Part model, mm, in its own coordinate system. A direction names the side the tool comes from. Give positions to 0.01 mm unless a question says otherwise; leave off trailing zeros. Answer as CSV lines item,"result". Start each with the question number.
1) Pin check, flat tips, straight feed: pin 1 Ø5 at (x, z) = (51.5, -35.5) entering from +Y; pin 2 Ø5 at (x, y) = (50, 102.5) entering from +Z; pin 3 Ø25 at (x, y) = (33, 62.5) entering from -Z. Stop position of each tip, or through.
2) Wall check: line 1 along X through (y, z) = (31, -4); line 2 along Z through (x, y) = (58.5, 97.5); line 3 along Y through (x, z) = (9, -16.5). Give the ranges that are in metal, low to high. Write a range as from..to.
3) Tool access for faces 1 (the flat face through (112.5, 45, -14)), 2 (the flat face through (57, 77, -19.295)): list every direction of +Z, -Z, +X, -X, +Y, -Y with a clear straight run to the whole face (end or side of a thin tool).
Autodesk Inventor part; units mm, degrees
ref_plane "Work Plane4" through (0, 100, 0) normal (0, 0.7071068, 0.7071068) x (1, 0, 0)
ref_plane "YZ Plane" through (0, 0, 0) normal (1, 0, 0) x (0, 1, 0)
ref_plane "XZ Plane" through (0, 0, 0) normal (0, 1, 0) x (-1, 0, 0)
sketch "Sketch1" plane through (0, 0, 0) normal (0, 0, 1) x (1, 0, 0)
  arc A0 (12.7973, -6.8176) -> (-12.597, -7.1809) centre (0, 0) ccw
  arc A1 (50.4829, -6.2785) -> (26.2017, -6.6259) centre (38.25, 0) ccw
  arc A2 (85.5853, -5.7763) -> (63.5844, -6.091) centre (74.5, 0) ccw
  arc A3 (117.8988, -5.314) -> (98.5072, -5.5914) centre (108.125, 0) ccw
  arc A4 (147.9764, -4.8837) -> (130.6669, -5.1313) centre (139.25, 0) ccw
  arc A5 (177.1345, -4.4665) -> (160.4967, -4.7045) centre (168.75, 0) ccw
  line L0 (-20, 20) -> (188.75, 20)
  line L1 (188.75, 20) -> (188.75, -4.3003)
  line L2 (-20, 20) -> (-20, -7.2868)
  line L3 (-20, -7.2868) -> (188.75, -4.3003)
  dimension "d0" = 29
  dimension "d1" = 27.5
  dimension "d2" = 25
  dimension "d3" = 22.25
  dimension "d4" = 20
  dimension "d5" = 19
  dimension "d6" = 38.25
  dimension "d7" = 36.25
  dimension "d8" = 33.625
  dimension "d9" = 31.125
  dimension "d10" = 29.5
  dimension "d11" = 0
  dimension "d12" = 0
  dimension "d13" = 0
  dimension "d14" = 0
  dimension "d15" = 0
  dimension "d20" = 20
  dimension "d22" = 20
  dimension "d23" = 20
  dimension "d24" = 7
  dimension "d25" = 4.586
sketch "Sketch4" plane through (0, 0, 0) normal (1, 0, 0) x (0, 1, 0)
  line L0 (0, 0) -> (29.9033, -29.9033)
  line L1 (0, 5.9807) -> (0, -35.884)
  point P0 (100, 0)
  dimension "d51" = 45
  dimension "d53" = 0
  dimension "d55" = 29.9033
  dimension "d98" = 100
ref_plane "Work Plane4" through (0, 100, 0) normal (0, 0.7071068, 0.7071068) x (1, 0, 0)
ref_plane "Work Plane3" through (-10, 0, 0) normal (0, 0.7071068, 0.7071068) x (1, 0, 0)
sketch "Sketch5" plane through (-10, 0, 0) normal (0, 0.7071068, 0.7071068) x (1, 0, 0)
  arc A0 (42.7973, 0.4692) -> (17.403, 0.1059) centre (30, 7.2868) ccw
  arc A1 (80.4829, 1.0084) -> (56.2017, 0.661) centre (68.25, 7.2868) ccw
  arc A2 (115.5853, 1.5106) -> (93.5844, 1.1958) centre (104.5, 7.2868) ccw
  arc A3 (147.8988, 1.9729) -> (128.5072, 1.6954) centre (138.125, 7.2868) ccw
  arc A4 (177.9764, 2.4032) -> (160.6669, 2.1555) centre (169.25, 7.2868) ccw
  arc A5 (207.1345, 2.8203) -> (190.4967, 2.5823) centre (198.75, 7.2868) ccw
  line L0 (10, 27.2868) -> (218.75, 27.2868)
  line L1 (218.75, 27.2868) -> (218.75, 2.9865)
  line L2 (10, 27.2868) -> (10, 0)
  line L3 (10, 0) -> (17.403, 0.1059)
  line L4 (42.7973, 0.4692) -> (56.2017, 0.661)
  line L5 (80.4829, 1.0084) -> (93.5844, 1.1958)
  line L6 (115.5853, 1.5106) -> (128.5072, 1.6954)
  line L7 (207.1345, 2.8203) -> (218.75, 2.9865)
  line L8 (147.8988, 1.9729) -> (160.6669, 2.1555)
  line L9 (177.9764, 2.4032) -> (190.4967, 2.5823)
  dimension "d56" = 29
  dimension "d57" = 27.5
  dimension "d58" = 25
  dimension "d59" = 22.25
  dimension "d60" = 20
  dimension "d61" = 19
  dimension "d62" = 38.25
  dimension "d63" = 36.25
  dimension "d64" = 33.625
  dimension "d65" = 31.125
  dimension "d66" = 29.5
  dimension "d67" = 0
  dimension "d68" = 0
  dimension "d69" = 0
  dimension "d70" = 0
  dimension "d71" = 0
  dimension "d72" = 20
  dimension "d73" = 20
  dimension "d74" = 20
sketch "Sketch6" plane through (0, 100, 0) normal (0, 0.7071068, 0.7071068) x (1, 0, 0)
  arc A0 (32.7973, 0.4692) -> (7.403, 0.1059) centre (20, 7.2868) ccw
  arc A1 (70.4829, 1.0084) -> (46.2017, 0.661) centre (58.25, 7.2868) ccw
  arc A2 (105.5853, 1.5106) -> (83.5844, 1.1958) centre (94.5, 7.2868) ccw
  arc A3 (137.8988, 1.9729) -> (118.5072, 1.6954) centre (128.125, 7.2868) ccw
  arc A4 (167.9764, 2.4032) -> (150.6669, 2.1555) centre (159.25, 7.2868) ccw
  arc A5 (197.1345, 2.8203) -> (180.4967, 2.5823) centre (188.75, 7.2868) ccw
  line L0 (0, 27.2868) -> (208.75, 27.2868)
  line L1 (208.75, 27.2868) -> (208.75, 2.9865)
  line L2 (0, 27.2868) -> (0, 0)
  line L3 (0, 0) -> (7.403, 0.1059)
  line L4 (32.7973, 0.4692) -> (46.2017, 0.661)
  line L5 (70.4829, 1.0084) -> (83.5844, 1.1958)
  line L6 (105.5853, 1.5106) -> (118.5072, 1.6954)
  line L7 (137.8988, 1.9729) -> (150.6669, 2.1555)
  line L8 (167.9764, 2.4032) -> (180.4967, 2.5823)
  line L9 (197.1345, 2.8203) -> (208.75, 2.9865)
  point P0 (0, -70.7107)
  dimension "d77" = 29
  dimension "d78" = 27.5
  dimension "d79" = 25
  dimension "d80" = 22.25
  dimension "d81" = 20
  dimension "d82" = 19
  dimension "d83" = 38.25
  dimension "d84" = 36.25
  dimension "d85" = 33.625
  dimension "d86" = 31.125
  dimension "d87" = 29.5
  dimension "d88" = 0
  dimension "d89" = 0
  dimension "d90" = 0
  dimension "d91" = 0
  dimension "d92" = 0
  dimension "d93" = 20
  dimension "d94" = 20
  dimension "d95" = 20
loft "Loft1" add profiles "Sketch6", "Sketch5"
sketch "Sketch7" plane through (0, 0, 0) normal (0, 1, 0) x (-1, 0, 0)
  line L0 (0, 0) -> (0, -19.2947)
  line L1 (0, -19.2947) -> (-208.75, -19.2947)
  line L2 (-208.75, -19.2947) -> (-208.75, -2.1118)
  line L3 (-208.75, -2.1118) -> (-197.1345, -1.9943)
  ellipse E0 centre (-188.75, -5.1526) end of major axis (-198.25, -5.1526) minor radius 6.7175 (-197.1345, -1.9943) -> (-180.4967, -1.826) ccw
  line L4 (-180.4967, -1.826) -> (-167.9764, -1.6993)
  ellipse E1 centre (-159.25, -5.1526) end of major axis (-169.25, -5.1526) minor radius 7.0711 (-167.9764, -1.6993) -> (-150.6669, -1.5242) ccw
  line L5 (-150.6669, -1.5242) -> (-137.8988, -1.395)
  ellipse E2 centre (-128.125, -5.1526) end of major axis (-139.25, -5.1526) minor radius 7.8666 (-137.8988, -1.395) -> (-118.5072, -1.1989) ccw
  line L6 (-118.5072, -1.1989) -> (-105.5853, -1.0681)
  ellipse E3 centre (-94.5, -5.1526) end of major axis (-107, -5.1526) minor radius 8.8388 (-105.5853, -1.0681) -> (-83.5844, -0.8456) ccw
  line L7 (-83.5844, -0.8456) -> (-70.4829, -0.713)
  ellipse E4 centre (-58.25, -5.1526) end of major axis (-72, -5.1526) minor radius 9.7227 (-70.4829, -0.713) -> (-46.2017, -0.4674) ccw
  line L8 (-46.2017, -0.4674) -> (-32.7973, -0.3318)
  ellipse E5 centre (-20, -5.1526) end of major axis (-34.5, -5.1526) minor radius 10.253 (-32.7973, -0.3318) -> (-7.403, -0.0749) ccw
  line L9 (-7.403, -0.0749) -> (0, 0)
  line L10 (0, 0) -> (0, -19.2947)
  line L11 (0, -19.2947) -> (-208.75, -19.2947)
  line L12 (-208.75, -19.2947) -> (-208.75, -2.1118)
  line L13 (-208.75, -2.1118) -> (0, 0)
sketch "Sketch10" plane through (0, 19.2947, -19.2947) normal (-1, 0, 0) x (0, 0, 1)
  line L0 (19.2947, 80.7053) -> (0, 100)
  line L1 (0, 100) -> (0, 0)
  line L2 (19.2947, -19.2947) -> (0, 0)
  line L3 (19.2947, 80.7053) -> (19.2947, -19.2947)
  line L4 (19.2947, -19.2947) -> (19.2947, -24.2947)
  line L5 (0, 0) -> (0, -22.6066)
  line L6 (0, -22.6066) -> (19.2947, -24.2947)
  line L7 (0, -22.6066) -> (-24.9049, -20.4278)
  line L8 (-24.9049, -20.4278) -> (0, 17.5461)
  line L9 (0, 100) -> (0, 0)
  line L10 (0, 17.5461) -> (0, 0)
  point P0 (19.2947, -19.2947)
  dimension "d106" = 5
  dimension "d111" = 85
  dimension "d113" = 25
  dimension "d114" = 40
sketch "Sketch11" plane through (208.75, 2.1118, -2.1118) normal (1, 0, 0) x (0, 0, -1)
  line L0 (17.1829, 117.1829) -> (0, 100)
  line L1 (0, 100) -> (0, 0)
  line L2 (17.1829, 17.1829) -> (0, 0)
  line L3 (17.1829, 117.1829) -> (17.1829, 17.1829)
  line L4 (17.1829, 17.1829) -> (0, 0)
  line L5 (10.1119, 10.1119) -> (-0.5876, -0.5876)
  line L6 (17.1829, -5.4237) -> (-2.1118, -7.1118)
  line L7 (0, 0) -> (0, -6.927)
  line L8 (17.1829, -5.4237) -> (0, -6.927)
  line L9 (17.1829, -5.4237) -> (17.1829, 17.1829)
  line L10 (0, -6.927) -> (17.1829, -5.4237)
  line L11 (17.1829, -5.4237) -> (42.0878, -3.2448)
  line L12 (42.0878, -3.2448) -> (17.1829, 34.5763)
  line L13 (17.1829, 117.1829) -> (17.1829, 17.1829)
  line L14 (17.1829, 17.1829) -> (17.1829, 34.5763)
  point P0 (-2.1118, -2.1118)
  point P1 (17.1829, -7.1118)
  point P2 (-0.4125, -0.4125)
  dimension "d115" = 25
  dimension "d116" = 40
loft "Loft3" add profiles "Sketch10", "Sketch11" contours L4 L6 L5 L2 | L1 L5 L7 L8 / L12 L11 L9 L3 | L2 L9 L6 L7
sketch "Sketch13" plane through (0, -1.133, -44.1996) normal (0, -0.9961947, -0.0871557) x (1, 0, 0)
  line L0 (0, 35.2171) -> (0, 14.3141)
  line L1 (7.403, 35.1359) -> (0, 35.2171)
  ellipse E0 centre (20, 29.635) end of major axis (5.5, 29.635) minor radius 11.1076 (7.403, 35.1359) -> (32.7973, 34.8576) ccw
  line L2 (46.2017, 34.7107) -> (32.7973, 34.8576)
  ellipse E1 centre (58.25, 29.635) end of major axis (44.5, 29.635) minor radius 10.5331 (46.2017, 34.7107) -> (70.4829, 34.4446) ccw
  line L3 (83.5844, 34.301) -> (70.4829, 34.4446)
  ellipse E2 centre (94.5, 29.635) end of major axis (82, 29.635) minor radius 9.5756 (83.5844, 34.301) -> (105.5853, 34.0599) ccw
  line L4 (118.5072, 33.9183) -> (105.5853, 34.0599)
  ellipse E3 centre (128.125, 29.635) end of major axis (117, 29.635) minor radius 8.5222 (118.5072, 33.9183) -> (137.8988, 33.7058) ccw
  line L5 (150.6669, 33.5658) -> (137.8988, 33.7058)
  ellipse E4 centre (159.25, 29.635) end of major axis (149.25, 29.635) minor radius 7.6604 (150.6669, 33.5658) -> (167.9764, 33.3761) ccw
  line L6 (180.4967, 33.2389) -> (167.9764, 33.3761)
  ellipse E5 centre (188.75, 29.635) end of major axis (179.25, 29.635) minor radius 7.2774 (180.4967, 33.2389) -> (197.1345, 33.0566) ccw
  line L7 (208.75, 32.9293) -> (197.1345, 33.0566)
  line L8 (208.75, 14.3141) -> (208.75, 32.9293)
  line L9 (0, 14.3141) -> (208.75, 14.3141)
  line L10 (0, 0) -> (0, 44.3684)
  line L11 (0, 0) -> (208.75, 0)
  line L12 (208.75, 0) -> (208.75, 42.2486)
  line L13 (0, 44.3684) -> (208.75, 42.2486)
  line L14 (0, 0) -> (208.75, 0)
  line L15 (112.5, 0) -> (112.5, 43.226)
  point P0 (0, 43.9326)
  dimension "d122" = 18
split body "Split1" sketch "Sketch13" result one side removed curves L15 removed pieces at (176.6667, 64.2471, -18.7947)
properties part number "coin_holder_large_only"
Found:
1,pin 1,"y = 15.93"
1,pin 2,"z = -11.21"
1,pin 3,"z = -19.29"
2,line 1,"0..5.59, 34.41..44.6, 71.9..82.11, 106.89..112.5"
2,line 2,"-19.29..-14.87"
2,line 3,"-3.56..116.5"
3,face 1,"+Z, -Z, +X, +Y, -Y"
3,face 2,"-Z, +X, -X, +Y"
